The listing builds one solid part. Answer for the finished solid, in the listing's coordinates (mm). A direction names the side the tool comes from. Coordinates: 2 decimals unless noted, no trailing zeros. Loops run counter-clockwise (first coordinate to the right, second up) from the corner with the lowest first, then second, coordinate; pieces in that order, holes last. Notation, with made-up numbers: M 32,31 L 49,31 A19 cw 49,59 Z; hole C 46,64.5 d2. An arc over 180 degrees is marked long. Return JSON: item names as keys, results as strings. Group by question number.
1. Section D-D (z = -1.5) is taken. Write down the section's boundary in (x, y).
2. Straight lines are drawn through the part: L1, parallel to Y at x = 0, z = 2.6; L2, parallel to Z at x = 1.25, y = 4; L3, parallel to Z at x = 9, y = 7.25. For each, find the intervals that lie inside material, in ascending order. Write a range as from..to.
3. The mould has two halves that part along Y. Classify faces 1 (the face through (-14.985, 0.66, 1.479)), 2 (the face through (-6.814, -3.135, 2.754)), 3 (the face through (0, 12, -7)), 4 (the face through (5.5, 1, 2.8)): pulls with the +Y half, pulls with the -Y half, needs draft (parallel to the pull), parting line crosses it, or undercut.
4. Given P1, Ø4, axis at y = -10, z = 1.5, coming from the +X side; P2, Ø0.6, axis at x = 5, z = 3, coming from the +Y side; P3, Ø0.6, axis at x = -10, z = 3, coming from the -Y side, each flat-ended and moving along its own axis, determine where each tip first touches the part or whether it passes through.
5. Section C-C (z = 1) is taken. Write down the section's boundary in (x, y), then the cut area to 3 significant figures.
6. Section B-B (y = -12) is taken. Write down the section's boundary in (x, z), then the cut area to 3 significant figures.
7. Which of the six approach directions +Z, -Z, +X, -X, +Y, -Y give full straight-line access (tool end or side, diameter ignored) to faces 5 (the face through (-0.325, 10.536, -3.549)), 6 (the face through (9.54, 4.39, 2.75)), 7 (the face through (-1.5, 0.07, 1.48))?
```python
from build123d import *

# Parameters (mm, degrees)
CROQUIS1_R              = 15
CROQUIS1_R_2            = 1.5
SALIENTE_EXTRUIR1_DEPTH = 3
SALIENTE_EXTRUIR2_START = -10
CROQUIS2_R              = 1.5
SALIENTE_EXTRUIR2_DEPTH = 10
CORTAR_EXTRUIR1_DEPTH   = 0.5


with BuildPart() as part:
    # Croquis1 → Saliente-Extruir1 (new body)
    with BuildSketch(Plane.XY):
        Circle(CROQUIS1_R)
        with Locations((0, 12)):
            Circle(CROQUIS1_R_2, mode=Mode.SUBTRACT)
        with Locations((0, -12)):
            Circle(CROQUIS1_R_2, mode=Mode.SUBTRACT)
        Circle(CROQUIS1_R_2, mode=Mode.SUBTRACT)
    extrude(amount=SALIENTE_EXTRUIR1_DEPTH)

    # Croquis2 → Saliente-Extruir2 (add)
    with BuildSketch(Plane.XY.offset(3).offset(SALIENTE_EXTRUIR2_START)):
        with Locations((0, -12)):
            Circle(CROQUIS2_R)
        with Locations((0, 12)):
            Circle(CROQUIS2_R)
    extrude(amount=SALIENTE_EXTRUIR2_DEPTH)

    # Croquis3 → Cortar-Extruir1 (cut)
    with BuildSketch(Plane.XY.offset(3)):
        with BuildLine():
            Line((-7.424621202, -7.424621202), (-8.838834765, -8.838834765))
            ThreePointArc((-8.838834765, -8.838834765), (11.548494156, 4.783542905), (-12.5, 0))
            Line((-12.5, 0), (-13.5, 0))
            Line((-13.5, 0), (-11.5, -2))
            Line((-11.5, -2), (-9.5, 0))
            Line((-9.5, 0), (-10.5, 0))
            ThreePointArc((-10.5, 0), (9.700735091, 4.01817604), (-7.424621202, -7.424621202))
        make_face()
        with BuildLine():
            Line((5.5, 0), (4.5, 0))
            Line((4.5, 0), (6.5, 2))
            Line((6.5, 2), (8.5, 0))
            Line((8.5, 0), (7.5, 0))
            ThreePointArc((7.5, 0), (-6.929096494, -2.870125743), (5.303300859, 5.303300859))
            Line((5.303300859, 5.303300859), (3.889087297, 3.889087297))
            ThreePointArc((3.889087297, 3.889087297), (-5.081337429, -2.104758878), (5.5, 0))
        make_face()
    extrude(amount=-CORTAR_EXTRUIR1_DEPTH, mode=Mode.SUBTRACT)


solid = part.part
```
Worked out:
{
 "1": {"outline": "C 0,-12 d3; C 0,12 d3"},
 "2": {"L1": "-15..-12.5, -10.5..-7.5, -5.5..-1.5, 1.5..5.5, 7.5..10.5, 12.5..15", "L2": "0..3", "L3": "0..2.5"},
 "3": {"face 1": "parting line crosses it", "face 2": "undercut", "face 3": "needs draft", "face 4": "undercut"},
 "4": {"P1": "x = 12.69", "P2": "y = 14.24", "P3": "y = -11.44"},
 "5": {"outline": "C 0,0 d30; hole C 0,0 d3", "area": "700 mm^2"},
 "6": {"outline": "M -9,0 L -1.5,0 L -1.5,-7 L 1.5,-7 L 1.5,0 L 9,0 L 9,3 L 3.5,3 L 3.5,2.5 L -3.5,2.5 L -3.5,3 L -9,3 Z", "area": "71.5 mm^2"},
 "7": {"face 5": "-Z", "face 6": "+Z", "face 7": "+Z, -Z"}
}
